Source: CAD feature listing. Evaluate the final solid. Frame: model axes, mm. Coordinates: 2 decimals unless noted, no trailing zeros. Loops run counter-clockwise (first coordinate to the right, second up) from the corner with the lowest first, then second, coordinate; pieces in that order, holes last.
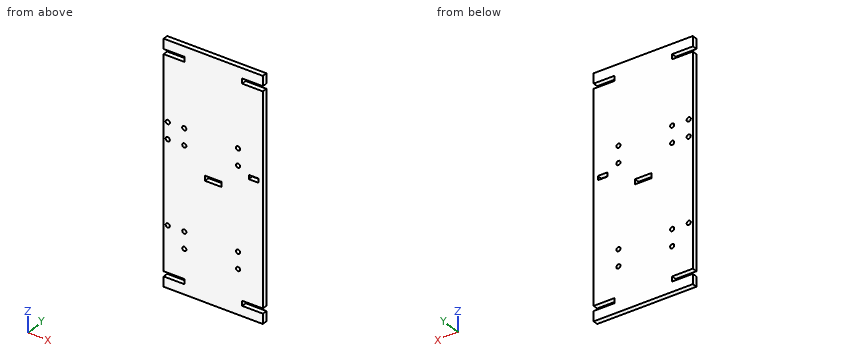
```python
from build123d import *

# Parameters (mm, degrees)
SKETCH1_W            = 120
SKETCH1_H            = 288
BOSS_EXTRUDE1_DEPTH  = 6
SKETCH2_W            = 25
SKETCH2_H            = 6
CUT_EXTRUDE1_DEPTH   = 313.057686975
LPATTERN1_COUNT      = 2
LPATTERN1_PITCH      = 258
LPATTERN1_COUNT_DIR2 = 2
LPATTERN1_PITCH_DIR2 = 95
SKETCH3_W            = 20
SKETCH3_H            = 6
CUT_EXTRUDE2_DEPTH   = 10
SKETCH4_R            = 2.5
CUT_EXTRUDE4_DEPTH   = 10
SKETCH6_W            = 12
SKETCH6_H            = 5
CUT_EXTRUDE5_DEPTH   = 10


with BuildPart() as part:
    # Sketch1 → Boss-Extrude1 (new body)
    with BuildSketch(Plane(origin=(0, 0, 0), x_dir=(1, 0, 0), z_dir=(0, 1, 0))):
        with Locations((-60, 144)):
            Rectangle(SKETCH1_W, SKETCH1_H)
    extrude(amount=BOSS_EXTRUDE1_DEPTH)

    # Sketch2 → Cut-Extrude1 (cut, through all)
    with BuildSketch(Plane(origin=(0, 6, 0), x_dir=(1, 0, 0), z_dir=(0, 1, 0))):
        with Locations((-107.5, 273)):
            Rectangle(SKETCH2_W, SKETCH2_H)
    cut_extrude1 = extrude(amount=-CUT_EXTRUDE1_DEPTH, mode=Mode.SUBTRACT)

    # LPattern1: Cut-Extrude1 2 × 2
    with Locations(*[(j * LPATTERN1_PITCH_DIR2, 0, i * LPATTERN1_PITCH) for i in range(LPATTERN1_COUNT) for j in range(LPATTERN1_COUNT_DIR2) if (i, j) != (0, 0)]):
        add(cut_extrude1, mode=Mode.SUBTRACT)

    # Sketch3 → Cut-Extrude2 (cut)
    with BuildSketch(Plane(origin=(0, 6, 0), x_dir=(1, 0, 0), z_dir=(0, 1, 0))):
        with Locations((-60, 144)):
            Rectangle(SKETCH3_W, SKETCH3_H)
    extrude(amount=-CUT_EXTRUDE2_DEPTH, mode=Mode.SUBTRACT)

    # Sketch4 → Cut-Extrude4 (cut)
    with BuildSketch(Plane(origin=(0, 6, 0), x_dir=(1, 0, 0), z_dir=(0, 1, 0))):
        with Locations(Location((-30, 235, 0), (0, 0, 270))):
            Circle(SKETCH4_R)
        with Locations(Location((-30, 215, 0), (0, 0, 270))):
            Circle(SKETCH4_R)
        with Locations(Location((-95, 235, 0), (0, 0, 270))):
            Circle(SKETCH4_R)
        with Locations(Location((-95, 215, 0), (0, 0, 270))):
            Circle(SKETCH4_R)
        with Locations(Location((-115, 215, 0), (0, 0, 270))):
            Circle(SKETCH4_R)
        with Locations(Location((-95, 115, 0), (0, 0, 270))):
            Circle(SKETCH4_R)
        with Locations(Location((-115, 115, 0), (0, 0, 270))):
            Circle(SKETCH4_R)
        with Locations(Location((-95, 95, 0), (0, 0, 270))):
            Circle(SKETCH4_R)
        with Locations(Location((-30, 115, 0), (0, 0, 270))):
            Circle(SKETCH4_R)
        with Locations(Location((-30, 95, 0), (0, 0, 270))):
            Circle(SKETCH4_R)
        with Locations(Location((-115, 95, 0), (0, 0, 270))):
            Circle(SKETCH4_R)
    extrude(amount=-CUT_EXTRUDE4_DEPTH, mode=Mode.SUBTRACT)

    # Sketch6 → Cut-Extrude5 (cut)
    with BuildSketch(Plane(origin=(0, 6, 0), x_dir=(1, 0, 0), z_dir=(0, 1, 0))):
        with Locations((-11, 123.5)):
            Rectangle(SKETCH6_W, SKETCH6_H)
    extrude(amount=-CUT_EXTRUDE5_DEPTH, mode=Mode.SUBTRACT)


solid = part.part
```
Q1. Section query B-B on z = -235. Return the cut outline in (x, y).
Q2. First-contact query: pin 1 Ø4 at (x, z) = (-30, -115) entering from +Y. Flat tip, straight axial feed; report the tip coordinate or a pass-through.
Q3. Material intervals for line 1 along X through (y, z) = (4.65, -215); line 2 along Z through (x, y) = (-101.5, 2); line 3 along Z through (x, y) = (-16, 5), sorted ascending.
Q4. Section query A-A on x = -14.5. Return the cut outline in (y, z).
Q5. Section query C-C on y = 3. Count the separate pieces of the cut face and the enclosed holes in it, then the cut area to 3 significant figures.
Resolved:
1. outline: (-120, 0) - (-97.5, 0) - (-97.5, 6) - (-120, 6) - close; (-92.5, 0) - (-32.5, 0) - (-32.5, 6) - (-92.5, 6) - close; (-27.5, 0) - (0, 0) - (0, 6) - (-27.5, 6) - close
2. pin 1: passes through
3. line 1: x = -120 to -117.5, -112.5 to -97.5, -92.5 to -32.5, -27.5 to 0
3. line 2: z = -288 to -276, -270 to -18, -12 to 0
3. line 3: z = -288 to -276, -270 to -126, -121 to -18, -12 to 0
4. outline: (0, -288) - (6, -288) - (6, -276) - (0, -276) - close; (0, -270) - (6, -270) - (6, -126) - (0, -126) - close; (0, -121) - (6, -121) - (6, -18) - (0, -18) - close; (0, -12) - (6, -12) - (6, 0) - (0, 0) - close
5. separate pieces: 1
5. enclosed holes: 13
5. area: 33,600 mm2
